For this review, use the dimensioned drawing (mm, ordinates from the lowest corner) and the shaded views. A direction names the side the tool comes from. Round coordinates to 2 decimals unless told otherwise and drop trailing zeros. Write each loop counter-clockwise with the first axis right and the second up, starting at its lowest first coordinate (ties: lowest second). Pieces come first, ordered by that corner, then holes. Notation, with made-up numbers: (-21, -34.75) - (-1, -34.75) arc R12 ccw to (-1, -30.75) - close; hole circle Ø1 at (62, 6). An arc over 180 degrees is marked (long way). Write each question's results on one line, items separated by ' | '.
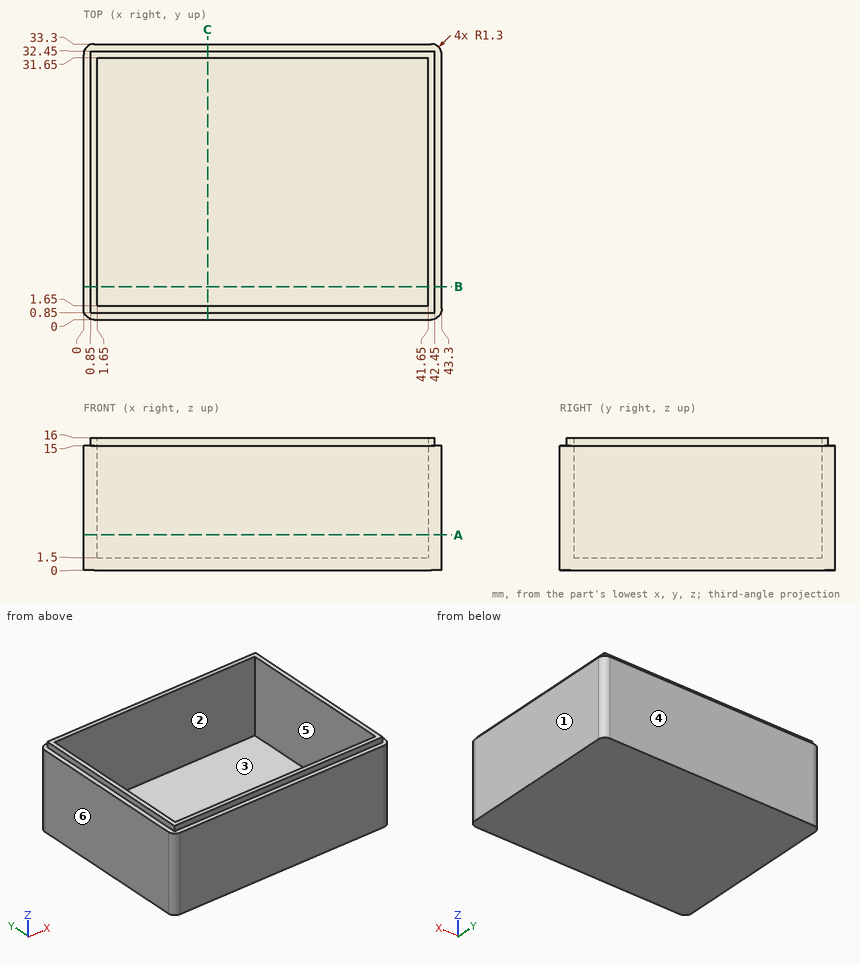
Q1. Tool access review of the marked faces 5 and 6: name each direction out of +Z, -Z, +X, -X, +Y, -Y from which nothing blocks a thin tool from reaching the whole face with its end or side.
Evaluation:
face 5: +Z | face 6: +Z, -Z, -X, +Y, -Y
Q2. Insertion check: P1, Ø0.8, axis at y = 24, z = 15.5, coming from the -X side; P2, Ø0.8, axis at y = 12.5, z = 15.5, coming from the +X side; P3, Ø0.5, axis at x = 21, z = 15.5, coming from the -Y side. Each pin has a flat end and moves straight along its axis. Give the tip position at first contact, or say it passes through.
Evaluation:
P1: stops at x = 0.85 | P2: stops at x = 42.45 | P3: stops at y = 0.85
Q3. We need section C-C (x = 15). State the section outline as (y, z) points.
Evaluation:
outline: (0, 0) - (33.3, 0) - (33.3, 15) - (32.45, 15) - (32.45, 16) - (31.65, 16) - (31.65, 1.5) - (1.65, 1.5) - (1.65, 16) - (0.85, 16) - (0.85, 15) - (0, 15) - close
Q4. We need section A-A (z = 4.25). State the section outline as (x, y) points, plus the area to 3 significant figures.
Evaluation:
outline: (0, 1.3) arc R1.3 ccw to (1.3, 0) - (42, 0) arc R1.3 ccw to (43.3, 1.3) - (43.3, 32) arc R1.3 ccw to (42, 33.3) - (1.3, 33.3) arc R1.3 ccw to (0, 32) - close; hole (1.65, 1.65) - (41.65, 1.65) - (41.65, 31.65) - (1.65, 31.65) - close | area: 240 mm^2
Q5. We need section B-B (y = 4). State the section outline as (x, z) points.
Evaluation:
outline: (0, 0) - (43.3, 0) - (43.3, 15) - (42.45, 15) - (42.45, 16) - (41.65, 16) - (41.65, 1.5) - (1.65, 1.5) - (1.65, 16) - (0.85, 16) - (0.85, 15) - (0, 15) - close
Q6. For probe 1 along X at (y, z) = (17.5, 2.75); probe 2 along Y at (x, z) = (37.5, 9); probe 3 along Z at (x, y) = (10.5, 9), list the stretches that pass through material, from the lowest coordinate up.
Evaluation:
probe 1: x = 0 to 1.65, 41.65 to 43.3 | probe 2: y = 0 to 1.65, 31.65 to 33.3 | probe 3: z = 0 to 1.5
Q7. The part is to be moulded in two halves that separate along X. For the marked faces 1, 2, 3 and 4, say which applies: released by +X, released by -X, zero draft, split by the parting line, or undercut.
Evaluation:
face 1: released by +X | face 2: undercut | face 3: undercut | face 4: zero draft
